from build123d import *

# Parameters (mm, degrees)
F1_DEPTH  = 2
F3_DEPTH  = 14.08
F4_DEPTH  = 10.425
F6_DEPTH  = 4
F8_DEPTH  = 0.345
F9_R      = 2.225
F10_DEPTH = 8
F11_R     = 1.95
F12_DEPTH = 2
F14_DEPTH = 2
F16_R     = 3
F17_DEPTH = 25


with BuildPart() as f1:
    # F0 (on Top) → F1 (new body)
    with BuildSketch(Plane.XY):
        with BuildLine():
            Line((-14.08, -8.11), (0, -8.11))
            Line((0, -8.11), (0, 0))
            Line((0, 0), (0, 8.11))
            Line((0, 8.11), (-14.08, 8.11))
            ThreePointArc((-14.08, 8.11), (-22.19, 0), (-14.08, -8.11))
        make_face()
    extrude(amount=F1_DEPTH)

    # F2 (on Right) → F3 (join)
    with BuildSketch(Plane.YZ):
        with BuildLine():
            Line((-8.11, 8.21), (-8.11, 2))
            Line((-8.11, 2), (8.11, 2))
            Line((8.11, 2), (8.11, 8.21))
            Line((8.11, 8.21), (3.4687412656, 21.99766178))
            ThreePointArc((3.4687412656, 21.99766178), (0, 24.49), (-3.4687412656, 21.99766178))
            Line((-3.4687412656, 21.99766178), (-8.11, 8.21))
        make_face()
    extrude(amount=-F3_DEPTH)

    # F4 (cut): a face of the model
    f4_faces = [f1.faces().sort_by_distance(p)[0] for p in [
        (0, 0, 10.1553909867),
    ]]
    extrude(f4_faces, amount=-F4_DEPTH, mode=Mode.SUBTRACT)

    # F5 (on face) → F6 (join)
    with BuildSketch(Plane(origin=(-14.08, 0, 0), x_dir=(0, -1, 0), z_dir=(-1, 0, 0))):
        with BuildLine():
            ThreePointArc((-3.4687412656, 21.99766178), (-0.5916109228, 17.2181311602), (3.66, 20.83))
            ThreePointArc((3.66, 20.83), (3.6118688398, 21.4216109228), (3.4687412656, 21.99766178))
            ThreePointArc((3.4687412656, 21.99766178), (0, 24.49), (-3.4687412656, 21.99766178))
        make_face()
    extrude(amount=F6_DEPTH)

    # F7 (on face) → F8 (join)
    with BuildSketch(Plane.YZ.offset(-10.425)):
        with BuildLine():
            ThreePointArc((-3.4687412656, 21.99766178), (-0.5916109228, 17.2181311602), (3.66, 20.83))
            ThreePointArc((3.66, 20.83), (3.6118688398, 21.4216109228), (3.4687412656, 21.99766178))
            ThreePointArc((3.4687412656, 21.99766178), (0, 24.49), (-3.4687412656, 21.99766178))
        make_face()
    extrude(amount=F8_DEPTH)

    # F9 (on face) → F10 (cut)
    with BuildSketch(Plane(origin=(-18.08, 0, 0), x_dir=(0, -1, 0), z_dir=(-1, 0, 0))):
        with Locations((0, 20.83)):
            Circle(F9_R)
    extrude(amount=-F10_DEPTH, mode=Mode.SUBTRACT)

    # F11 (on face) → F12 (cut)
    with BuildSketch(Plane.XY.offset(2)):
        with Locations((-17.265, 0)):
            Circle(F11_R)
    extrude(amount=-F12_DEPTH, mode=Mode.SUBTRACT)

    # F13 (on face) → F14 (join)
    with BuildSketch(Plane.XY):
        Polygon((-10.425, 8.11), (-10.425, -8.11), (0, -8.11), (0, 0), (0, 8.11), align=None)
    extrude(amount=F14_DEPTH)

    # F15: F1 across plane


with BuildPart() as f1_1:
    add(f1.part)
    add(f1.part.mirror(Plane.YZ))

    # F16 (on face) → F17 (cut)
    with BuildSketch(Plane.YZ.offset(14.08)):
        with Locations((0, 8.5717271108)):
            Circle(F16_R)
    extrude(amount=-F17_DEPTH, mode=Mode.SUBTRACT)


solid = f1_1.part
Could you check a few things on this model? Use its own coordinates, in mm. A direction names the side the tool comes from. Coordinates: 2 decimals unless noted, no trailing zeros. Order: outer loops, then holes, each group sorted by start corner. A loop starts at its lowest first (then second) coordinate and runs counter-clockwise, first axis right, second up.
Q1. Suppose I cut it at D-D on y = 4.25. Please give me the cut outline in (x, z) (3 decimals).
Q2. Please list where these lines run through material, in increasing order: L1, parallel to Z at x = 15, y = 0 (3 decimals); L2, parallel to Z at x = -10.6, y = 0 (3 decimals); L3, parallel to X at y = -0.75, z = 16.5 (3 decimals).
Q3. Will these pins go through, and if not, where does the flat tip stop? pin 1 (1 mm diameter, centred on y = 2, z = 14.5, fed in from -X); pin 2 (8 mm diameter, centred on y = -3.5, z = 15, fed in from -X); pin 3 (3.5 mm diameter, centred on x = 17.265, y = 0, fed in from -Z); pin 4 (4 mm diameter, centred on y = 0, z = 20.83, fed in from -X).
Q4. Suppose I cut it at C-C on x = 0. Please give me the cut outline in (y, z).
Q5. Suppose I cut it at B-B on y = 0. Give the number of separate pieces and of enclosed holes in the cut face, and give its area (3 significant figures).
Q6. Suppose I cut it at A-A on z = 10. Please give me the cut outline in (x, y) (3 decimals), and give its area (3 significant figures).
Q7. Which directions (+Z, -Z, +X, -X, +Y, -Y) give clear straight access to the entire face, cutting with the end or side of a thin tool? Please do faces 4 (the flat face through (18.08, -2, 19)), 5 (the flat face through (-18.08, -2, 19)), 6 (the flat face through (-10.08, 2, 19)), 7 (the cylindrical face through (12.28, -2.21, 10.6)).
Q8. Thinking about a two-plate mould opening in Z: for faces 1 (the flat face through (-18, 2, 2)), 2 (the flat face through (-12.23, 5.82, 15.01)), 3 (the flat face through (0, -8.11, 1)), which applies, released by +Z, released by -Z, zero draft, split by the parting line, or undercut?
Answer:
1. outline: (-20.987, 0) - (20.987, 0) - (20.987, 2) - (14.08, 2) - (14.08, 19.677) - (10.425, 19.677) - (10.425, 2) - (-10.425, 2) - (-10.425, 19.677) - (-14.08, 19.677) - (-14.08, 2) - (-20.987, 2) - close
2. L1: z = 0 to 2, 17.17 to 18.605, 23.055 to 24.49
2. L2: z = 0 to 5.572, 11.572 to 18.605, 23.055 to 24.49
2. L3: x = -14.08 to -10.425, 10.425 to 14.08
3. pin 1: stops at x = -14.08
3. pin 2: stops at x = -18.08
3. pin 3: stops at z = 17.17
3. pin 4: passes through
4. outline: (-8.11, 0) - (8.11, 0) - (8.11, 2) - (-8.11, 2) - close
5. separate pieces: 6
5. enclosed holes: 0
5. area: 205 mm2
6. outline: (-14.08, -7.507) - (-10.425, -7.507) - (-10.425, -2.638) - (-10.92, -2.638) - (-10.92, 2.638) - (-10.425, 2.638) - (-10.425, 7.507) - (-14.08, 7.507) - close; (10.425, -7.507) - (14.08, -7.507) - (14.08, -2.638) - (10.425, -2.638) - close; (10.425, 2.638) - (14.08, 2.638) - (14.08, 7.507) - (10.425, 7.507) - close
6. area: 87.9 mm2
7. face 4: +Z, +X, +Y, -Y
7. face 5: +Z, -X, +Y, -Y
7. face 6: +Z, +Y, -Y
7. face 7: +X
8. face 1: undercut
8. face 2: released by +Z
8. face 3: zero draft
